Design review of the part built by this model. Coordinates are the model's own, in mm. A direction names the side the tool comes from. Coordinates: 2 decimals unless noted, no trailing zeros. Loops run counter-clockwise (first coordinate to the right, second up) from the corner with the lowest first, then second, coordinate; pieces in that order, holes last. Notation, with made-up numbers: (31, 3) -> (71, 3) arc R30 cw to (71, 28) -> close; hole circle Ø5 at (63.5, 26.5). An arc over 180 degrees is marked (long way). Answer as a JSON object with one key per item and string values.
Autodesk Inventor part; units mm, degrees
ref_plane "YZ Plane" through (0, 0, 0) normal (1, 0, 0) x (0, 1, 0)
ref_plane "XZ Plane" through (0, 0, 0) normal (0, 1, 0) x (-1, 0, 0)
ref_plane "XY Plane" through (0, 0, 0) normal (0, 0, 1) x (1, 0, 0)
sketch "Sketch1" plane through (0, 0, 0) normal (0, 0, 1) x (1, 0, 0)
  line L0 (90.8, 43.3229) -> (90.8, 46.4979)
  line L1 (90.8, 46.4979) -> (100.8, 46.4979)
  line L2 (100.8, 46.4979) -> (100.8, 43.175)
  line L3 (94.45, 28.3229) -> (94.45, 18.3229)
  line L4 (90.8, 0.1479) -> (100.8, 0.1479)
  line L5 (100.8, 0.1479) -> (100.8, 6.35)
  line L6 (100.8, 6.35) -> (100.8, 18.3229)
  line L7 (94.45, 18.3229) -> (100.8, 18.3229)
  line L8 (100.8, 28.3229) -> (94.45, 28.3229)
  line L9 (100.8, 28.3229) -> (100.8, 43.175)
  line L10 (90.8, 3.3229) -> (90.8, 0.1479)
  line L11 (10, 3.3229) -> (90.8, 3.3229)
  line L12 (90.8, 43.3229) -> (10, 43.3229)
  line L13 (10, 43.3229) -> (10, 46.4979)
  line L14 (10, 46.4979) -> (0, 46.4979)
  line L15 (0, 46.4979) -> (0, 43.175)
  line L16 (10, 3.3229) -> (10, 0.1479)
  line L17 (6.35, 28.3229) -> (6.35, 18.3229)
  line L18 (0, 43.175) -> (0, 28.3229)
  line L19 (0, 28.3229) -> (6.35, 28.3229)
  line L20 (0, 18.3229) -> (0, 6.35)
  line L21 (6.35, 18.3229) -> (0, 18.3229)
  line L22 (0, 0.1479) -> (0, 6.35)
  line L23 (10, 0.1479) -> (0, 0.1479)
  line L24 (40.4, 20.8229) -> (60.4, 20.8229)
  line L25 (60.4, 20.8229) -> (60.4, 12.8229)
  line L26 (60.4, 12.8229) -> (40.4, 12.8229)
  line L27 (40.4, 12.8229) -> (40.4, 20.8229)
  line L28 (50.4, 43.3229) -> (50.4, 3.3229)
  point P0 (0, 0)
  point P1 (4.5679, 28.3229)
  point P2 (50.4, 12.8229)
  point P3 (6.35, 23.3229)
  point P4 (50.4, 23.3229)
  point P5 (94.45, 23.3229)
  dimension "d0" = 40
  dimension "d1" = 20
  dimension "d2" = 8
  dimension "d3" = 88.1
  dimension "d4" = 80.8
  dimension "d5" = 3.175
  dimension "d6" = 3.175
  dimension "d7" = 3.175
  dimension "d8" = 3.175
  dimension "d9" = 10
  dimension "d10" = 10
  dimension "d11" = 9.5
extrude "Extrusion1" add sketch "Sketch1" along normal blind 6.35
extrude "Extrusion2" cut sketch "Sketch1" along normal blind 6.35 contours L28 L26 L27 L24 | L24 L25 L26 L28
properties part number "boxBack"
1) Add section D-D, the plane x = 26. Give the boundary of the cut face in (y, z).
Completed:
{"outline": "(3.32, 0) -> (43.32, 0) -> (43.32, 6.35) -> (3.32, 6.35) -> close"}
2) Add section A-A, the plane x = 48. Give the boundary of the cut face in (y, z), and give its area (3 significant figures).
Completed:
{"outline": "(3.32, 0) -> (12.82, 0) -> (12.82, 6.35) -> (3.32, 6.35) -> close; (20.82, 0) -> (43.32, 0) -> (43.32, 6.35) -> (20.82, 6.35) -> close", "area": "203 mm²"}
3) Add section C-C, the plane z = 5.25. Give the boundary of the cut face in (x, y), and give its area (3 significant figures).
Completed:
{"outline": "(0, 0.15) -> (10, 0.15) -> (10, 3.32) -> (90.8, 3.32) -> (90.8, 0.15) -> (100.8, 0.15) -> (100.8, 18.32) -> (94.45, 18.32) -> (94.45, 28.32) -> (100.8, 28.32) -> (100.8, 46.5) -> (90.8, 46.5) -> (90.8, 43.32) -> (10, 43.32) -> (10, 46.5) -> (0, 46.5) -> (0, 28.32) -> (6.35, 28.32) -> (6.35, 18.32) -> (0, 18.32) -> close; hole (40.4, 12.82) -> (60.4, 12.82) -> (60.4, 20.82) -> (40.4, 20.82) -> close", "area": "3,870 mm²"}
4) The part is to be moulded in two halves that separate along X. For faces 5 (the flat face through (10, 45, 3)), 6 (the flat face through (0, 9, 3)), 7 (the flat face through (100.8, 38, 3)), 8 (the flat face through (50, 24, 0)), say which applies: pulls with the +X half, pulls with the -X half, needs draft (parallel to the pull), parting line crosses it, or undercut.
Completed:
{"face 5": "undercut", "face 6": "pulls with the -X half", "face 7": "pulls with the +X half", "face 8": "needs draft"}
5) Wall thickness on probe 1 along Y at (x, z) = (59, 2.25); probe 2 along X at (y, z) = (14.5, 4.5); probe 3 along X at (y, z) = (2.5, 4.75): over which ranges is each line inside the solid? List them lowest first.
Completed:
{"probe 1": "3.32 to 12.82, 20.82 to 43.32", "probe 2": "0 to 40.4, 60.4 to 100.8", "probe 3": "0 to 10, 90.8 to 100.8"}
6) Add section B-B, the plane y = 15. Give the boundary of the cut face in (x, z).
Completed:
{"outline": "(0, 0) -> (40.4, 0) -> (40.4, 6.35) -> (0, 6.35) -> close; (60.4, 0) -> (100.8, 0) -> (100.8, 6.35) -> (60.4, 6.35) -> close"}
7) Clearance check with flat-ended pins moving along their axes: pin 1 Ø2.5 at (y, z) = (1.5, 1.5) entering from -X; pin 2 Ø1.9 at (x, z) = (50, 4.5) entering from -Y; pin 3 Ø1.9 at (x, z) = (42, 4.5) entering from +Y. State where each tip first meets the part, or that it passes through.
Completed:
{"pin 1": "x = 0", "pin 2": "y = 3.32", "pin 3": "y = 43.32"}
8) For faces 1 (the flat face through (60.4, 17, 3)), 2 (the flat face through (51, 43.323, 3)), 3 (the flat face through (3, 18.323, 3)), 4 (the flat face through (10, 2, 3)), list the 3-axis set-ups (+Z, -Z, +X, -X, +Y, -Y) from which the entire face can be reached by the end or side of a thin tool; tool diameter is ignored.
Completed:
{"face 1": "+Z, -Z", "face 2": "+Z, -Z, +Y", "face 3": "+Z, -Z, -X", "face 4": "+Z, -Z, -Y"}
